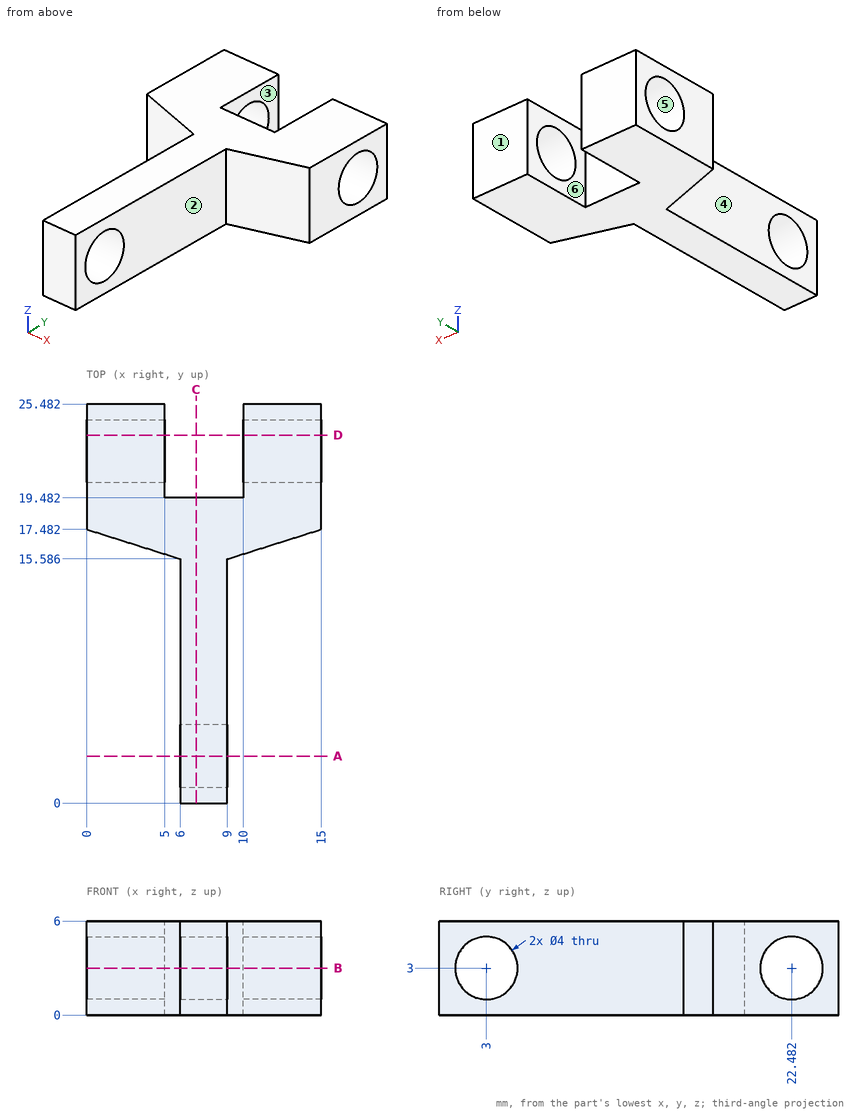
Check sheet for the drawn part. Datum: minimum x, y, z corner. Units: mm. A direction names the side the tool comes from. Round coordinates to 2 decimals unless told otherwise and drop trailing zeros. Loops run counter-clockwise (first coordinate to the right, second up) from the corner with the lowest first, then second, coordinate; pieces in that order, holes last. Notation, with made-up numbers: (-21.75, -25.5) - (1.25, -25.5) arc R20 ccw to (1.25, 4.5) - close; hole circle Ø10 at (14.25, 68.25). An arc over 180 degrees is marked (long way). Write each question's results on one line, items separated by ' | '. Start each with the question number.
Q1. Cross-section at D-D on y = 23.5. Enter the section's corners in (x, z).
Q2. Release check for a two-part mould opening along X. For the marked faces 4, 5 and 6 record: +X half, -X half, draft (parallel to the pull), parting line (faces both ways), or undercut.
Q3. Gauge pin test, flat ends, axial feed: P1, Ø2, axis at x = 7, z = 5, coming from the +Y side; P2, Ø3, axis at y = 6.5, z = 1, coming from the +X side; P3, Ø3.5, axis at y = 22.48, z = 3, coming from the +X side; P4, Ø3, axis at y = 11, z = 3, coming from the -X side. Record the tip position at first contact, or that the pin passes through.
Q4. Cross-section at A-A on y = 3. Enter the section's corners in (x, z).
Q5. Access from +Z, -Z, +X, -X, +Y, -Y to the whole of each face (thin tool, end or side, straight path). Record for the marked faces 1, 2 and 3.
Q6. Cross-section at B-B on z = 3. Enter the section's corners in (x, y).
Q7. Cross-section at C-C on x = 7. Enter the section's corners in (y, z).
Q8. Thickness scan on line 1 (X direction, y = 24.5, z = 5.4); line 2 (Z direction, x = 6.75, y = 3); line 3 (Y direction, x = 1, z = 2.15) (1 decimal). Record the ranges inside material, lowest first. Write a range as [from, to].
Answers below:
1) outline: (0, 0) - (5, 0) - (5, 1.28) - (0, 1.28) - close; (0, 4.72) - (5, 4.72) - (5, 6) - (0, 6) - close; (10, 0) - (15, 0) - (15, 1.28) - (10, 1.28) - close; (10, 4.72) - (15, 4.72) - (15, 6) - (10, 6) - close
2) face 4: -X half | face 5: draft | face 6: undercut
3) P1: stops at y = 19.48 | P2: stops at x = 9 | P3: passes through | P4: stops at x = 6
4) outline: (6, 0) - (9, 0) - (9, 1) - (6, 1) - close; (6, 5) - (9, 5) - (9, 6) - (6, 6) - close
5) face 1: +Z, -Z, +X, -X, +Y | face 2: +Z, -Z, +X, -Y | face 3: +Z, -Z, +Y
6) outline: (0, 17.48) - (6, 15.59) - (6, 5) - (9, 5) - (9, 15.59) - (15, 17.48) - (15, 20.48) - (10, 20.48) - (10, 19.48) - (5, 19.48) - (5, 20.48) - (0, 20.48) - close; (0, 24.48) - (5, 24.48) - (5, 25.48) - (0, 25.48) - close; (6, 0) - (9, 0) - (9, 1) - (6, 1) - close; (10, 24.48) - (15, 24.48) - (15, 25.48) - (10, 25.48) - close
7) outline: (0, 0) - (19.48, 0) - (19.48, 6) - (0, 6) - close; hole circle Ø4 at (3, 3)
8) line 1: x = [0, 5], [10, 15] | line 2: z = [0, 1], [5, 6] | line 3: y = [17.2, 20.7], [24.3, 25.5]
